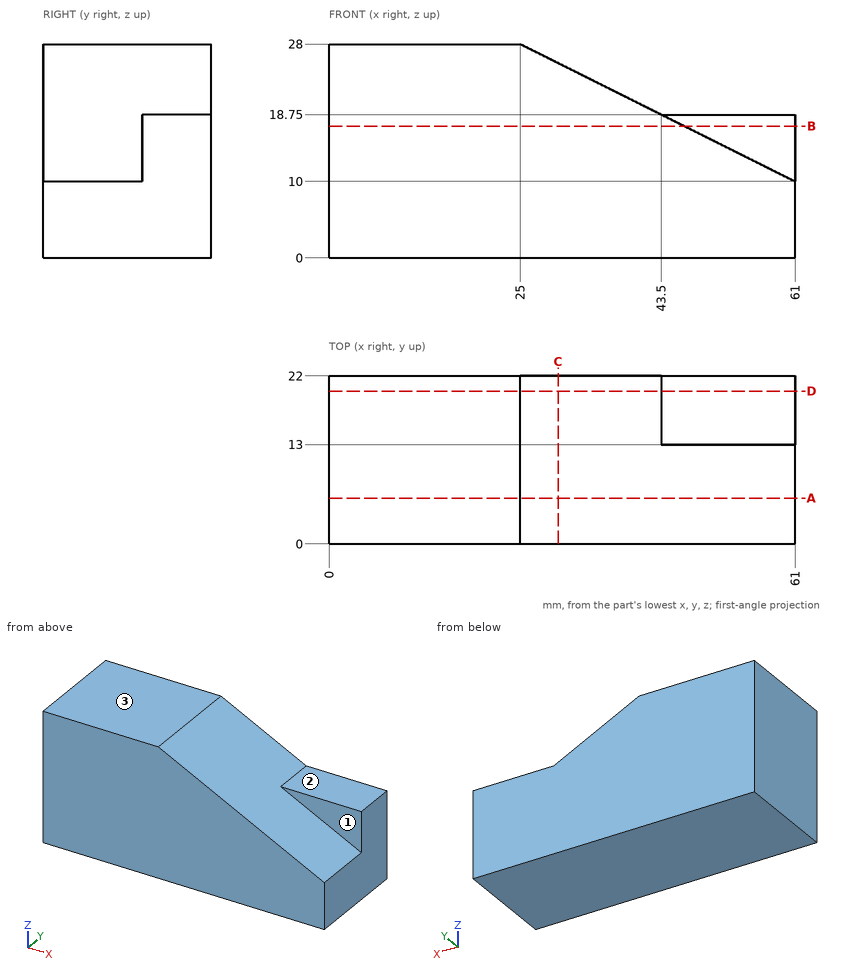
Part print with two shaded views. Sizes in mm from the minimum x, y, z corner. A direction names the side the tool comes from. Round coordinates to 2 decimals unless told otherwise and drop trailing zeros. Write each loop counter-clockwise with the first axis right and the second up, starting at its lowest first coordinate (ties: lowest second). Pieces come first, ordered by that corner, then holes. Notation, with made-up numbers: M 63.25,80 L 120.25,80 A19 cw 120.25,94 Z; hole C 75.5,-34.5 d1. An arc over 180 degrees is marked long. Use CSV: the item, a comma, the result in double quotes.
1. Saw through at C-C (x = 30). Give the cut face in (y, z), plus the area to 3 significant figures.
Reply:
outline,"M 0,0 L 22,0 L 22,25.5 L 0,25.5 Z"
area,"561 mm²"
2. Tool access for the marked faces 1, 2 and 3: list every direction of +Z, -Z, +X, -X, +Y, -Y with a clear straight run to the whole face (end or side of a thin tool).
Reply:
face 1,"+Z, +X, -Y"
face 2,"+Z, +X, +Y, -Y"
face 3,"+Z, +X, -X, +Y, -Y"
3. Wall check: probe 1 along Z at (x, y) = (47.5, 21.25); probe 2 along X at (y, z) = (11.5, 24.5); probe 3 along X at (y, z) = (6.25, 13). Give the ranges that are in metal, low to high. Write a range as from..to.
Reply:
probe 1,"z = 0..18.75"
probe 2,"x = 0..32"
probe 3,"x = 0..55"
4. Flat gauge pins, fed straight in: pin 1 (8 mm diameter, centred on x = 15, y = 12, fed in from -Z); pin 2 (10 mm diameter, centred on x = 56.5, y = 17, fed in from +Z); pin 3 (1.5 mm diameter, centred on x = 37.5, y = 13, fed in from +Z) (3 decimals). Where does each tip first touch, or does it go through?
Reply:
pin 1,"stops at z = 0"
pin 2,"stops at z = 18.75"
pin 3,"stops at z = 22.125"
5. Saw through at B-B (z = 17.25). Give the cut face in (x, y), plus the area to 3 significant figures.
Reply:
outline,"M 0,0 L 46.5,0 L 46.5,13 L 61,13 L 61,22 L 0,22 Z"
area,"1,150 mm²"
6. Saw through at A-A (y = 6). Give the cut face in (x, z), plus the area to 3 significant figures.
Reply:
outline,"M 0,0 L 61,0 L 61,10 L 25,28 L 0,28 Z"
area,"1,380 mm²"
7. Saw through at D-D (y = 20). Give the cut face in (x, z), plus the area to 3 significant figures.
Reply:
outline,"M 0,0 L 61,0 L 61,18.75 L 43.5,18.75 L 25,28 L 0,28 Z"
area,"1,460 mm²"
